Read the model definition and answer for the solid it produces. Units are mm, in the model's axes. A direction names the side the tool comes from. Coordinates: 2 decimals unless noted, no trailing zeros. Order: outer loops, then holes, each group sorted by start corner. A loop starts at its lowest first (then second) coordinate and runs counter-clockwise, first axis right, second up. Notation, with made-up numbers: (23, 11.5) -> (49, 11.5) arc R24 cw to (49, 42.5) -> close; hole circle Ø9 at (52, -20.75). An arc over 180 degrees is marked (long way). Answer as a JSON object with one key per item and string values. Group by question number.
1) A tool of negligible diameter and unlimited length cuts with its end or side. For faces 1 (the flat face through (0, -12.25, 12)), 2 (the flat face through (12.25, 0, 12)), 3 (the cylindrical face through (-0.325, -15.035, 7.464)), 4 (the flat face through (-15, 0, 11)), 5 (the flat face through (0, 12.25, 12)), from which of +Z, -Z, +X, -X, +Y, -Y can it reach the whole face along a straight path? Write none if from no direction.
2) Determine the mould class of faces 6 (the flat face through (0, -12.5, 6)), 7 (the cylindrical face through (-0.325, 15.035, 7.464)), 8 (the flat face through (-17.5, 0, 5)), 9 (the flat face through (17.5, 0, 5)) for opening direction X: released by +X, released by -X, zero draft, split by the parting line, or undercut.
3) Given pin 1 (4 mm diameter, centred on x = 7.5, z = 13.5, fed in from +Y); pin 2 (0.9 mm diameter, centred on x = -0.5, z = 6.5, fed in from -Y); pin 3 (1 mm diameter, centred on x = -12, y = 0, fed in from +Z), each flat-ended and moving along its own axis, determine where each tip first touches the part or whether it passes through.
4) Section B-B on y = 9.5 is taken. Determine the outline of the cut face in (x, z).
5) Section A-A on z = 6 is taken. Determine the outline of the cut face in (x, y), and give its area (3 significant figures).
6) Section D-D on y = 13.5 is taken. Determine the outline of the cut face in (x, z).
7) Consider L1, parallel to Z at x = 0, y = 15.35; L2, parallel to X at y = -16.1, z = 6; L3, parallel to Z at x = -13.5, y = 0. Determine where each line is inside the solid, lowest interval first.
from build123d import *

# Parameters (mm, degrees)
SKETCH1_W           = 35
SKETCH1_H           = 35
BOSS_EXTRUDE1_DEPTH = 11
SKETCH2_R           = 1.5
CUT_EXTRUDE1_DEPTH  = 5
SKETCH3_W           = 24.5
SKETCH3_H           = 24.5
BOSS_EXTRUDE2_DEPTH = 2.5
SKETCH4_R           = 7
BOSS_EXTRUDE3_DEPTH = 9
FILLET1_R           = 0.5
FILLET2_R           = 0.5


with BuildPart() as part:
    # Sketch1 → Boss-Extrude1 (new body)
    with BuildSketch(Plane.XY):
        Rectangle(SKETCH1_W, SKETCH1_H)
    extrude(amount=BOSS_EXTRUDE1_DEPTH)

    # Sketch2 → Cut-Extrude1 (cut)
    with BuildSketch(Plane(origin=(0, 17.5, 0), x_dir=(1, 0, 0), z_dir=(0, 1, 0))):
        with Locations((0, -6)):
            Circle(SKETCH2_R)
    cut_extrude1 = extrude(amount=-CUT_EXTRUDE1_DEPTH, mode=Mode.SUBTRACT)

    # Mirror1: Cut-Extrude1 across plane
    add(cut_extrude1.mirror(Plane.ZX), mode=Mode.SUBTRACT)

    # Sketch3 → Boss-Extrude2 (add)
    with BuildSketch(Plane.XY.offset(11)):
        Rectangle(SKETCH3_W, SKETCH3_H)
    extrude(amount=BOSS_EXTRUDE2_DEPTH)

    # Sketch4 → Boss-Extrude3 (add)
    with BuildSketch(Plane.XY.offset(13.5)):
        Circle(SKETCH4_R)
    extrude(amount=BOSS_EXTRUDE3_DEPTH)

    # Fillet1
    fillet1_edges = [part.edges().sort_by_distance(p)[0] for p in [
        (-17.5, 0, 11),
        (0, -17.5, 11),
        (12.25, -12.25, 12.25),
        (12.25, 12.25, 12.25),
        (-12.25, 12.25, 12.25),
        (-12.25, -12.25, 12.25),
        (12.25, 0, 13.5),
        (0, 12.25, 13.5),
        (-12.25, 0, 13.5),
        (0, -12.25, 13.5),
        (-7, 0, 13.5),
        (17.5, 0, 11),
        (0, -17.5, 0),
        (-17.5, 0, 0),
        (0, 17.5, 0),
        (17.5, 0, 0),
        (0, 17.5, 11),
        (17.5, -17.5, 5.5),
        (-17.5, -17.5, 5.5),
        (-17.5, 17.5, 5.5),
        (17.5, 17.5, 5.5),
    ]]
    fillet(fillet1_edges, radius=FILLET1_R)

    # Fillet2
    fillet2_edges = [part.edges().sort_by_distance(p)[0] for p in [
        (-7, 0, 22.5),
    ]]
    fillet(fillet2_edges, radius=FILLET2_R)


solid = part.part
Worked answers:
{
 "1": {"face 1": "+Z, +X, -X, -Y", "face 2": "+Z, +X, +Y, -Y", "face 3": "-Y", "face 4": "+Z", "face 5": "+Z, +X, -X, +Y"},
 "2": {"face 6": "undercut", "face 7": "undercut", "face 8": "released by -X", "face 9": "released by +X"},
 "3": {"pin 1": "stops at y = 12.25", "pin 2": "stops at y = -12.5", "pin 3": "stops at z = 13.5"},
 "4": {"outline": "(-17.5, 0.5) arc R0.5 ccw to (-17, 0) -> (17, 0) arc R0.5 ccw to (17.5, 0.5) -> (17.5, 10.5) arc R0.5 ccw to (17, 11) -> (12.25, 11) -> (12.25, 13) arc R0.5 ccw to (11.75, 13.5) -> (-11.75, 13.5) arc R0.5 ccw to (-12.25, 13) -> (-12.25, 11) -> (-17, 11) arc R0.5 ccw to (-17.5, 10.5) -> close"},
 "5": {"outline": "(-17.5, -17) arc R0.5 ccw to (-17, -17.5) -> (-1.5, -17.5) -> (-1.5, -12.5) -> (1.5, -12.5) -> (1.5, -17.5) -> (17, -17.5) arc R0.5 ccw to (17.5, -17) -> (17.5, 17) arc R0.5 ccw to (17, 17.5) -> (1.5, 17.5) -> (1.5, 12.5) -> (-1.5, 12.5) -> (-1.5, 17.5) -> (-17, 17.5) arc R0.5 ccw to (-17.5, 17) -> close", "area": "1,190 mm²"},
 "6": {"outline": "(-17.5, 0.5) arc R0.5 ccw to (-17, 0) -> (17, 0) arc R0.5 ccw to (17.5, 0.5) -> (17.5, 10.5) arc R0.5 ccw to (17, 11) -> (-17, 11) arc R0.5 ccw to (-17.5, 10.5) -> close; hole circle Ø3 at (0, 6)"},
 "7": {"L1": "z = 0 to 4.5, 7.5 to 11", "L2": "x = -17.5 to -1.5, 1.5 to 17.5", "L3": "z = 0 to 11"}
}
